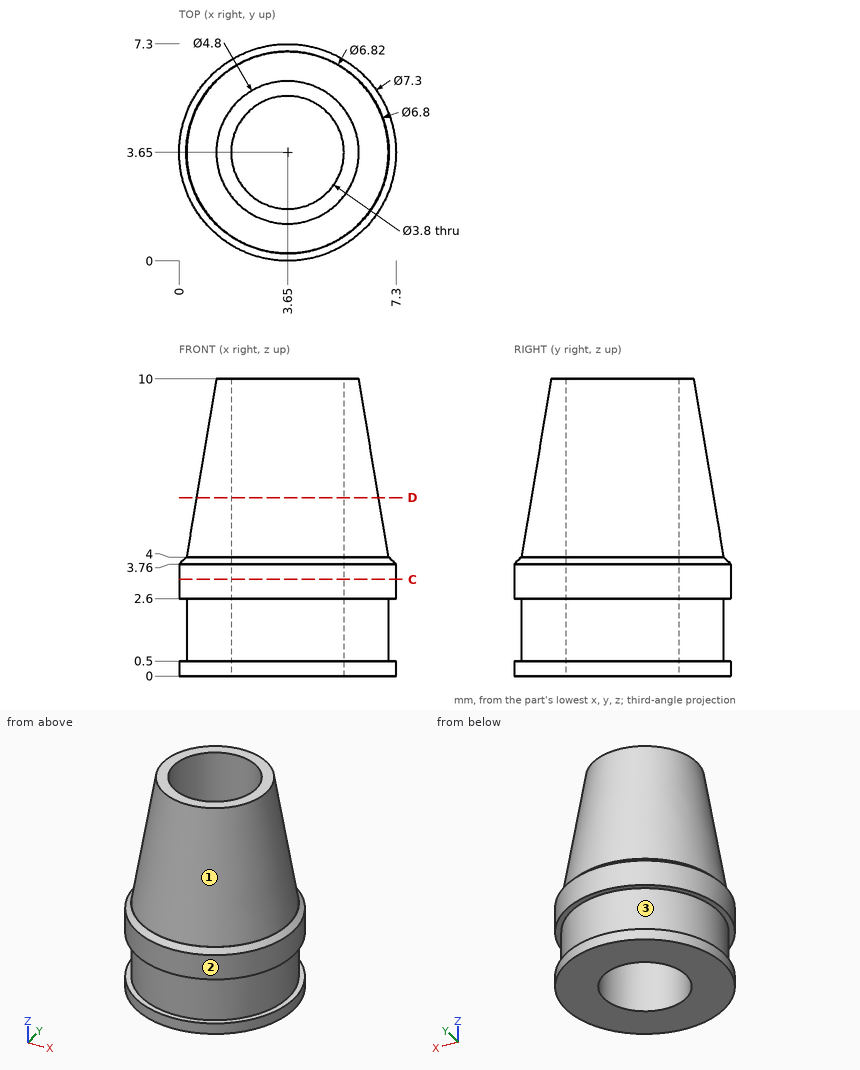
For this review, use the dimensioned drawing (mm, ordinates from the lowest corner) and the shaded views. Round coordinates to 2 decimals unless told otherwise and drop trailing zeros. Order: outer loops, then holes, each group sorted by start corner. A loop starts at its lowest first (then second) coordinate and runs counter-clockwise, first axis right, second up. Notation, with made-up numbers: (-24, -39.5) -> (-15, -39.5) arc R23 cw to (-15, -14.5) -> close; hole circle Ø8 at (52, -25). An arc over 180 degrees is marked (long way). Write item = value, one per line. Start each with the question number.
Item 1: Consider section C-C on z = 3.25. Write out the cut boundary in (x, y), plus the area to 3 significant figures.
Item 2: For line 1 along Y through (x, z) = (3.5, 5.5); line 2 along X through (y, z) = (4.25, 6); line 3 along Z through (x, y) = (1.5, 6.5), list the stretches that pass through material, from the lowest coordinate up.
Item 3: Clearance check with a flat-ended pin moving along its axis: pin 1 Ø1.5 at (x, y) = (5, 1) entering from -Z. State where the tip first meets the part, or that it passes through.
Item 4: Mouldability with a two-part tool opening along Z and no side actions: class the marked faces 1, 2 and 3 as released by +Z, released by -Z, zero draft, split by the parting line, or undercut.
Item 5: Consider section D-D on z = 6. Write out the cut boundary in (x, y), plus the area to 3 significant figures.
Conclusion:
q1.outline = circle Ø7.3 at (3.65, 3.65); hole circle Ø3.8 at (3.65, 3.65)
q1.area = 30.5 mm2
q2.line_1 = 0.5 to 1.76, 5.54 to 6.8
q2.line_2 = 0.64 to 1.85, 5.45 to 6.66
q2.line_3 = 0 to 0.5, 2.6 to 3.84
q3.pin_1 = 0
q4.face_1 = released by +Z
q4.face_2 = zero draft
q4.face_3 = undercut
q5.outline = circle Ø6.13 at (3.65, 3.65); hole circle Ø3.8 at (3.65, 3.65)
q5.area = 18.2 mm2
